Design review of the part built by this model. Coordinates are the model's own, in mm. A direction names the side the tool comes from. Coordinates: 2 decimals unless noted, no trailing zeros. Write each loop counter-clockwise with the first axis right and the second up, starting at its lowest first coordinate (ties: lowest second). Pieces come first, ordered by that corner, then holes. Notation, with made-up numbers: M 61.5,23 L 109.5,23 A12 ccw 109.5,46 Z; hole C -19.5,-33 d1. An arc over 180 degrees is marked long. One line per question, with ' | ' between items.
from build123d import *

# Parameters (mm, degrees)
SKETCH1_R           = 5
SKETCH1_R_2         = 2.75
BOSS_EXTRUDE1_DEPTH = 2
SKETCH2_W           = 10
SKETCH2_H           = 10
BOSS_EXTRUDE2_DEPTH = 15
SKETCH3_R           = 2.75
SKETCH3_W           = 20
SKETCH3_H           = 10
BOSS_EXTRUDE3_DEPTH = 5
SKETCH4_R           = 5
BOSS_EXTRUDE4_DEPTH = 12.5
SKETCH5_R           = 2.85
BOSS_EXTRUDE5_DEPTH = 52
BOSS_EXTRUDE6_START = 5
SKETCH6_R           = 2.75
BOSS_EXTRUDE6_DEPTH = 5
SKETCH8_R           = 2.75
BOSS_EXTRUDE7_DEPTH = 2


with BuildPart() as part:
    # Sketch1 → Boss-Extrude1 (new body)
    # profile 1 of 3: a face of its own
    with BuildSketch(Plane.XY):
        with Locations((-20, -30)):
            Circle(SKETCH1_R)
        with Locations((-20, -30)):
            Circle(SKETCH1_R_2, mode=Mode.SUBTRACT)
    # profile 2 of 3: a face of its own
    with BuildSketch(Plane.XY):
        with BuildLine():
            Line((20, -25), (-20, -25))
            ThreePointArc((-20, -25), (-16.464466094, -26.464466094), (-15, -30))
            ThreePointArc((-15, -30), (-16.464466094, -33.535533906), (-20, -35))
            Line((-20, -35), (20, -35))
            ThreePointArc((20, -35), (15, -30), (20, -25))
        make_face()
    # profile 3 of 3: a face of its own
    with BuildSketch(Plane.XY):
        with Locations((20, -30)):
            Circle(SKETCH1_R)
        with Locations((20, -30)):
            Circle(SKETCH1_R_2, mode=Mode.SUBTRACT)
    extrude(amount=BOSS_EXTRUDE1_DEPTH)

    # Sketch2 → Boss-Extrude2 (add)
    with BuildSketch(Plane.XY.offset(2)):
        with Locations((-5, -30)):
            Rectangle(SKETCH2_W, SKETCH2_H)
        with Locations((5, -30)):
            Rectangle(SKETCH2_W, SKETCH2_H)
    extrude(amount=BOSS_EXTRUDE2_DEPTH)

    # Sketch3 → Boss-Extrude3 (add)
    # profile 1 of 3: a face of its own
    with BuildSketch(Plane.XY.offset(17)):
        with BuildLine():
            Line((-10, -25), (-20, -25))
            ThreePointArc((-20, -25), (-25, -30), (-20, -35))
            Line((-20, -35), (-10, -35))
            Line((-10, -35), (-10, -25))
        make_face()
        with Locations((-20, -30)):
            Circle(SKETCH3_R, mode=Mode.SUBTRACT)
    # profile 2 of 3: a face of its own
    with BuildSketch(Plane.XY.offset(17)):
        with Locations((0, -30)):
            Rectangle(SKETCH3_W, SKETCH3_H)
    # profile 3 of 3: a face of its own
    with BuildSketch(Plane.XY.offset(17)):
        with BuildLine():
            Line((10, -35), (20, -35))
            ThreePointArc((20, -35), (25, -30), (20, -25))
            Line((20, -25), (10, -25))
            Line((10, -25), (10, -35))
        make_face()
        with Locations((20, -30)):
            Circle(SKETCH3_R, mode=Mode.SUBTRACT)
    extrude(amount=BOSS_EXTRUDE3_DEPTH)

    # Sketch4 → Boss-Extrude4 (add)
    with BuildSketch(Plane.XY.offset(22)):
        with Locations(Location((20, -30, 0), (0, 0, 180))):
            Circle(SKETCH4_R)
        with Locations(Location((-20, -30, 0), (0, 0, 180))):
            Circle(SKETCH4_R)
    extrude(amount=BOSS_EXTRUDE4_DEPTH)

    # Sketch5 → Boss-Extrude5 (add)
    with BuildSketch(Plane.XY.offset(34.5)):
        with Locations((20, -30)):
            Circle(SKETCH5_R)
        with Locations((-20, -30)):
            Circle(SKETCH5_R)
    extrude(amount=BOSS_EXTRUDE5_DEPTH)

    # Sketch6 → Boss-Extrude6 (add)
    with BuildSketch(Plane(origin=(0, 0, 22), x_dir=(-1, 0, 0), z_dir=(0, 0, -1)).offset(BOSS_EXTRUDE6_START)):
        with Locations(Location((20, -30, 0), (0, 0, 180))):
            Circle(SKETCH6_R)
        with Locations(Location((-20, -30, 0), (0, 0, 180))):
            Circle(SKETCH6_R)
    extrude(amount=-BOSS_EXTRUDE6_DEPTH)

    # Sketch8 → Boss-Extrude7 (add)
    # profile 1 of 2: a face of its own
    with BuildSketch(Plane.XY.offset(2)):
        with BuildLine():
            Line((-10, -35), (-10, -25))
            Line((-10, -25), (-20, -25))
            ThreePointArc((-20, -25), (-25, -30), (-20, -35))
            Line((-20, -35), (-10, -35))
        make_face()
        with Locations((-20, -30)):
            Circle(SKETCH8_R, mode=Mode.SUBTRACT)
    # profile 2 of 2: a face of its own
    with BuildSketch(Plane.XY.offset(2)):
        with BuildLine():
            Line((20, -25), (10, -25))
            Line((10, -25), (10, -35))
            Line((10, -35), (20, -35))
            ThreePointArc((20, -35), (25, -30), (20, -25))
        make_face()
        with Locations((20, -30)):
            Circle(SKETCH8_R, mode=Mode.SUBTRACT)
    extrude(amount=BOSS_EXTRUDE7_DEPTH)


solid = part.part
1. Draft analysis for pull direction X (two halves, no side actions). For faces 1 (the face through (0, -30, 0)), 2 (the face through (-22.747, -29.879, 1.972)), 3 (the face through (17.973, -28.141, 1.972)), 4 (the face through (-10, -30, 10)), state which applies: pulls with the +X half, pulls with the -X half, needs draft (parallel to the pull), parting line crosses it, or undercut.
Answer sheet:
face 1: needs draft | face 2: undercut | face 3: undercut | face 4: pulls with the -X half
2. Insertion check: pin 1 Ø3 at (x, y) = (-19, -30) entering from -Z; pin 2 Ø5 at (x, y) = (6.5, -29.5) entering from +Z; pin 3 Ø2 at (y, z) = (-27.5, 46) entering from -X. Each pin has a flat end and moves straight along its axis. Give the tip position at first contact, or say it passes through.
Answer sheet:
pin 1: z = 17 | pin 2: z = 22 | pin 3: x = -22.42
3. Take a section at D-D (z = 10.5). Write out the cut boundary in (x, y).
Answer sheet:
outline: M -10,-35 L 10,-35 L 10,-25 L -10,-25 Z
4. Take a section at A-A (x = 14). Write out the cut boundary in (y, z).
Answer sheet:
outline: M -35,0 L -25,0 L -25,4 L -35,4 Z; M -35,17 L -25,17 L -25,22 L -35,22 Z
5. To check wall thickness, follow line 1 along Y through (x, z) = (-20, 3); line 2 along X through (y, z) = (-29.25, 48.5); line 3 along Z through (x, y) = (22, -26.5). State the ranges of each line that lie inside material, in increasing order. Write a range as [from, to].
Answer sheet:
line 1: [-35, -32.75], [-27.25, -25] | line 2: [-22.75, -17.25], [17.25, 22.75] | line 3: [0, 4], [17, 34.5]
6. Tool access review of faces 5 (the face through (0, -25, 11)), 6 (the face through (-16, -30, 4)), 7 (the face through (10, -30, 10)), 8 (the face through (17.8, -27.8, 34.5)): name each direction out of +Z, -Z, +X, -X, +Y, -Y from which nothing blocks a thin tool from reaching the whole face with its end or side.
Answer sheet:
face 5: +Z, -Z, +X, -X, +Y | face 6: -X, +Y, -Y | face 7: +X, +Y, -Y | face 8: +Z
7. Take a section at C-C (x = 19). Write out the cut boundary in (y, z), then the cut area to 3 significant figures.
Answer sheet:
outline: M -35,0 L -32.56,0 L -32.56,4 L -35,4 Z; M -35,17 L -25,17 L -25,22 L -25.1,22 L -25.1,34.5 L -27.33,34.5 L -27.33,86.5 L -32.67,86.5 L -32.67,34.5 L -34.9,34.5 L -34.9,22 L -35,22 Z; M -27.44,0 L -25,0 L -25,4 L -27.44,4 Z | area: 470 mm^2
8. Take a section at B-B (y = -31.75). Count the separate pieces of the cut face and the enclosed holes in it, then the cut area to 3 significant figures.
Answer sheet:
separate pieces: 3 | enclosed holes: 0 | area: 1,370 mm^2
